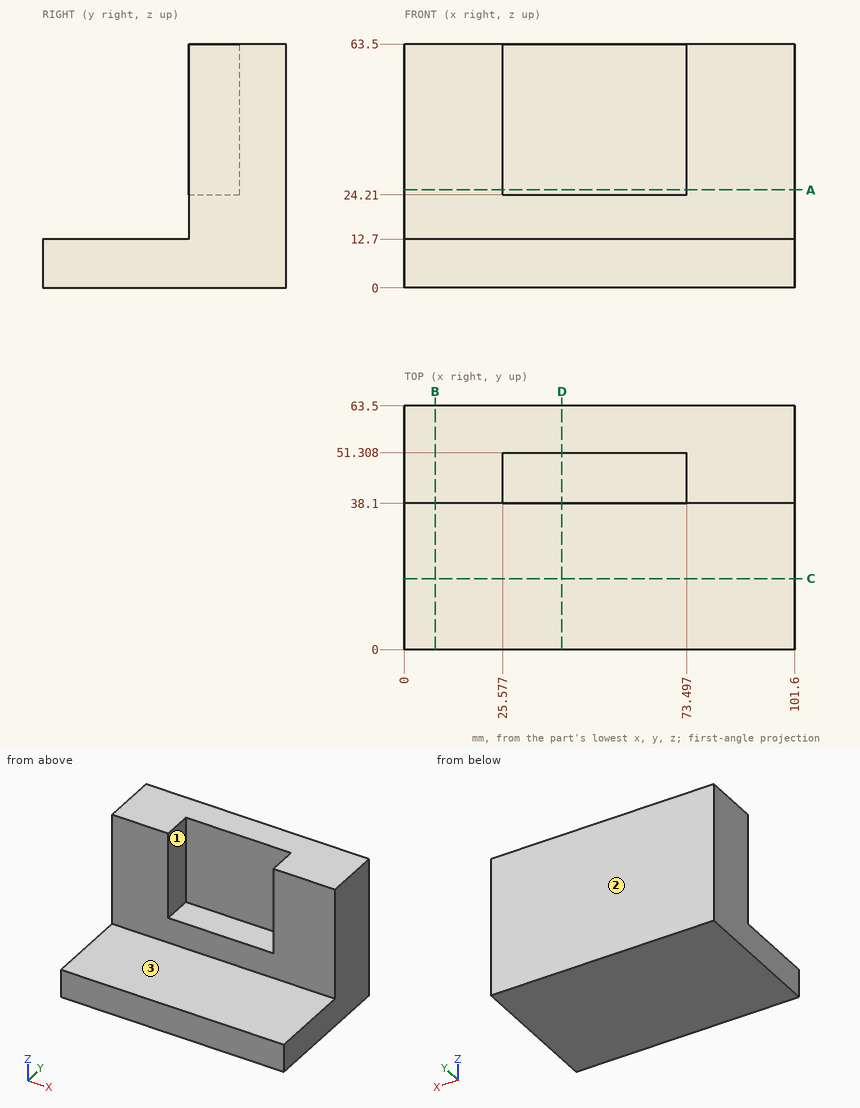
Here's the drawing with two shaded views (mm, measured from the low corner). I have some questions. A direction names the side the tool comes from. Coordinates: 2 decimals unless noted, no trailing zeros. Write each loop counter-clockwise with the first axis right and the second up, starting at its lowest first coordinate (ties: lowest second). Pieces come first, ordered by that corner, then holes. Notation, with made-up numbers: (43.25, -1.5) - (59.25, -1.5) arc R10 ccw to (59.25, 8.5) - close; hole circle Ø9 at (86.25, -6.75). An arc over 180 degrees is marked (long way). Return JSON: item names as keys, results as strings.
Q1. If we section it at B-B (x = 8): Please give me the cut outline in (y, z), then the cut area to 3 significant figures.
Computed values:
{"outline": "(0, 0) - (63.5, 0) - (63.5, 63.5) - (38.1, 63.5) - (38.1, 12.7) - (0, 12.7) - close", "area": "2,100 mm2"}
Q2. Please list where these lines run through material, in increasing order: L1, parallel to X at y = 47.5, z = 30.5; L2, parallel to Y at x = 93, z = 20.5; L3, parallel to Y at x = 39.5, z = 39.5. Write a range as from..to.
Computed values:
{"L1": "x = 0..25.58, 73.5..101.6", "L2": "y = 38.1..63.5", "L3": "y = 51.31..63.5"}
Q3. If we section it at C-C (y = 18.5): Please give me the cut outline in (x, z).
Computed values:
{"outline": "(0, 0) - (101.6, 0) - (101.6, 12.7) - (0, 12.7) - close"}
Q4. I'm going to push flat-ended pins straight in: pin 1 Ø12 at (y, z) = (43, 52) entering from -X; pin 2 Ø4 at (x, y) = (43, 43.5) entering from +Z; pin 3 Ø8 at (x, y) = (27, 31) entering from +Z. Where does each tip first touch, or does it pass through?
Computed values:
{"pin 1": "stops at x = 0", "pin 2": "stops at z = 24.21", "pin 3": "stops at z = 12.7"}
Q5. On a 3-axis mill with a long thin cutter (end or side, diameter ignored), from which of +Z, -Z, +X, -X, +Y, -Y can I reach the whole of each face in a straight line? I mean the marked faces 1, 2 and 3. Say none if no direction works.
Computed values:
{"face 1": "+Z, -Y", "face 2": "+Z, -Z, +X, -X, +Y", "face 3": "+Z, +X, -X, -Y"}
Q6. If we section it at A-A (z = 25.5): Please give me the cut outline in (x, y).
Computed values:
{"outline": "(0, 38.1) - (25.58, 38.1) - (25.58, 51.31) - (73.5, 51.31) - (73.5, 38.1) - (101.6, 38.1) - (101.6, 63.5) - (0, 63.5) - close"}
Q7. If we section it at D-D (x = 41): Please give me the cut outline in (y, z), then the cut area to 3 significant figures.
Computed values:
{"outline": "(0, 0) - (63.5, 0) - (63.5, 63.5) - (51.31, 63.5) - (51.31, 24.21) - (38.1, 24.21) - (38.1, 12.7) - (0, 12.7) - close", "area": "1,580 mm2"}
